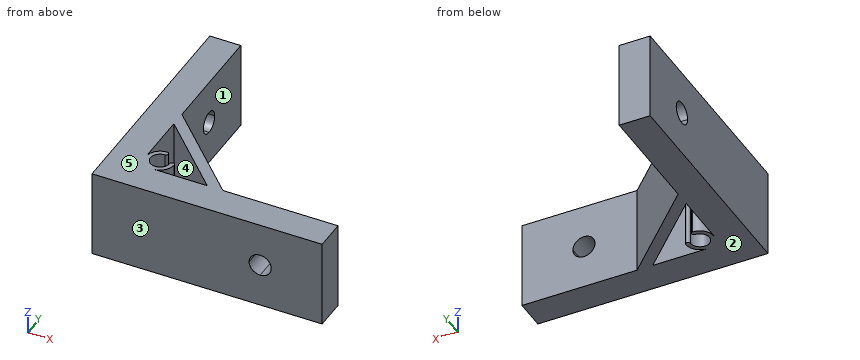
```python
from build123d import *

# Parameters (mm, degrees)
BOSS_EXTRUDE1_DEPTH = 20
CUT_EXTRUDE1_DEPTH  = 7


with BuildPart() as part:
    # Sketch1 → Boss-Extrude1 (new body)
    with BuildSketch(Plane.XY):
        Polygon((0, 52), (0, 0), (52, 0), (52, 7), (26, 7), (7, 26), (7, 52), align=None)
        with BuildLine():
            Line((7, 10.175), (7, 22.464466094))
            Line((7, 22.464466094), (22.464466094, 7))
            Line((22.464466094, 7), (10.175, 7))
            ThreePointArc((10.175, 7), (12.42006403, 7.92993597), (13.35, 10.175))
            ThreePointArc((13.35, 10.175), (12.85, 10.675), (12.35, 10.175))
            ThreePointArc((12.35, 10.175), (8.637042751, 8.637042751), (10.175, 12.35))
            ThreePointArc((10.175, 12.35), (10.675, 12.85), (10.175, 13.35))
            ThreePointArc((10.175, 13.35), (7.92993597, 12.42006403), (7, 10.175))
        make_face(mode=Mode.SUBTRACT)
    extrude(amount=BOSS_EXTRUDE1_DEPTH)

    # Sketch2 → Cut-Extrude1 (cut)
    with BuildSketch(Plane(origin=(7, 0, 0), x_dir=(0, 0, -1), z_dir=(1, 0, 0))):
        with BuildLine():
            ThreePointArc((-7.5, 38), (-8.232233047, 39.767766953), (-10, 40.5))
            Line((-10, 40.5), (-10, 35.5))
            ThreePointArc((-10, 35.5), (-8.232233047, 36.232233047), (-7.5, 38))
        make_face()
        with BuildLine():
            Line((-10, 35.5), (-10, 40.5))
            ThreePointArc((-10, 40.5), (-12.5, 38), (-10, 35.5))
        make_face()
    cut_extrude1 = extrude(amount=-CUT_EXTRUDE1_DEPTH, mode=Mode.SUBTRACT)

    # Mirror4: Cut-Extrude1 across plane
    add(cut_extrude1.mirror(Plane(origin=(0, 0, 0), x_dir=(0, 0, 1), z_dir=(0.7071067811865438, -0.7071067811865512, 0))), mode=Mode.SUBTRACT)


solid = part.part
```
Here's how the part is built. I have some questions about the finished solid (model axes, mm). Face numbers are marked on the shaded views. A direction names the side the tool comes from. Give positions to 0.01 mm unless a question says otherwise; leave off trailing zeros. Order: outer loops, then holes, each group sorted by start corner. A loop starts at its lowest first (then second) coordinate and runs counter-clockwise, first axis right, second up. Notation, with made-up numbers: (88.5, -36.5) -> (108.5, -36.5) arc R23 ccw to (108.5, -21.5) -> close; hole circle Ø1 at (-8, 28.5). An arc over 180 degrees is marked (long way). Use CSV: the item, a comma, the result in double quotes. Start each with the question number.
Item 1: On a 3-axis mill with a long thin cutter (end or side, diameter ignored), from which of +Z, -Z, +X, -X, +Y, -Y can I reach the whole of each face in a straight line? I mean the marked faces 1 and 2. Say none if no direction works.
Item 2: Suppose I cut it at C-C (x = 14). List the corners of the cut face in (y, z) for me.
Item 3: Thinking about a two-plate mould opening in Y: for the marked faces 3, 4 and 5, which applies, pulls with the +Y half, pulls with the -Y half, needs draft (parallel to the pull), parting line crosses it, or undercut?
Item 4: Suppose I cut it at A-A (y = 39.5). List the corners of the cut face in (x, z) for me.
Item 5: If I drill on probe 1 along X at (y, z) = (8.5, 8.75); probe 2 along X at (y, z) = (47, 10), over which ranges is the centre line in solid material (lowest first)? Write a range as [from, to].
Item 6: Suppose I cut it at D-D (y = 9.5). List the corners of the cut face in (x, z) for me.
Item 7: Suppose I cut it at B-B (z = 18). List the corners of the cut face in (x, y) for me (3 decimals), and give its area (3 significant figures).
Item 8: I'm going to push flat-ended pins straight in: P1, Ø12, axis at x = 42, z = 3.5, coming from the +Y side; P2, Ø4, axis at y = 42.5, z = 12, coming from the +X side; P3, Ø6, axis at y = 18, z = 8, coming from the +X side. Where does each tip first touch, or does it pass through?
Answer block:
1,face 1,"+Z, -Z, +X, +Y"
1,face 2,"-Z, +X, -X, +Y, -Y"
2,outline,"(0, 0) -> (7, 0) -> (7, 20) -> (0, 20) -> close; (15.46, 0) -> (19, 0) -> (19, 20) -> (15.46, 20) -> close"
3,face 3,"pulls with the -Y half"
3,face 4,"undercut"
3,face 5,"needs draft"
4,outline,"(0, 0) -> (7, 0) -> (7, 8) -> (0, 8) -> close; (0, 12) -> (7, 12) -> (7, 20) -> (0, 20) -> close"
5,probe 1,"x = [0, 8.79], [11.56, 12.87], [20.96, 24.5]"
5,probe 2,"x = [0, 7]"
6,outline,"(0, 0) -> (8.11, 0) -> (8.11, 20) -> (0, 20) -> close; (12.24, 0) -> (13.28, 0) -> (13.28, 20) -> (12.24, 20) -> close; (19.96, 0) -> (23.5, 0) -> (23.5, 20) -> (19.96, 20) -> close"
7,outline,"(0, 0) -> (52, 0) -> (52, 7) -> (26, 7) -> (7, 26) -> (7, 52) -> (0, 52) -> close; hole (7, 10.175) arc R3.175 cw to (10.175, 13.35) arc R0.5 cw to (10.175, 12.35) arc R2.175 ccw (long way) to (12.35, 10.175) arc R0.5 cw to (13.35, 10.175) arc R3.175 cw to (10.175, 7) -> (22.464, 7) -> (7, 22.464) -> close"
7,area,"755 mm^2"
8,P1,"stops at y = 7"
8,P2,"stops at x = 7"
8,P3,"stops at x = 18"
